For this review, use the dimensioned drawing (mm, ordinates from the lowest corner) and the shaded views. A direction names the side the tool comes from. Give positions to 0.01 mm unless a question says otherwise; leave off trailing zeros. Order: outer loops, then holes, each group sorted by start corner. A loop starts at its lowest first (then second) coordinate and runs counter-clockwise, first axis right, second up. Notation, with made-up numbers: (59, -20) -> (106, -20) arc R21 ccw to (106, 8) -> close; hole circle Ø7 at (84.25, 44). An arc over 180 degrees is marked (long way). Answer as a JSON object with one key per item and string values. Group by question number.
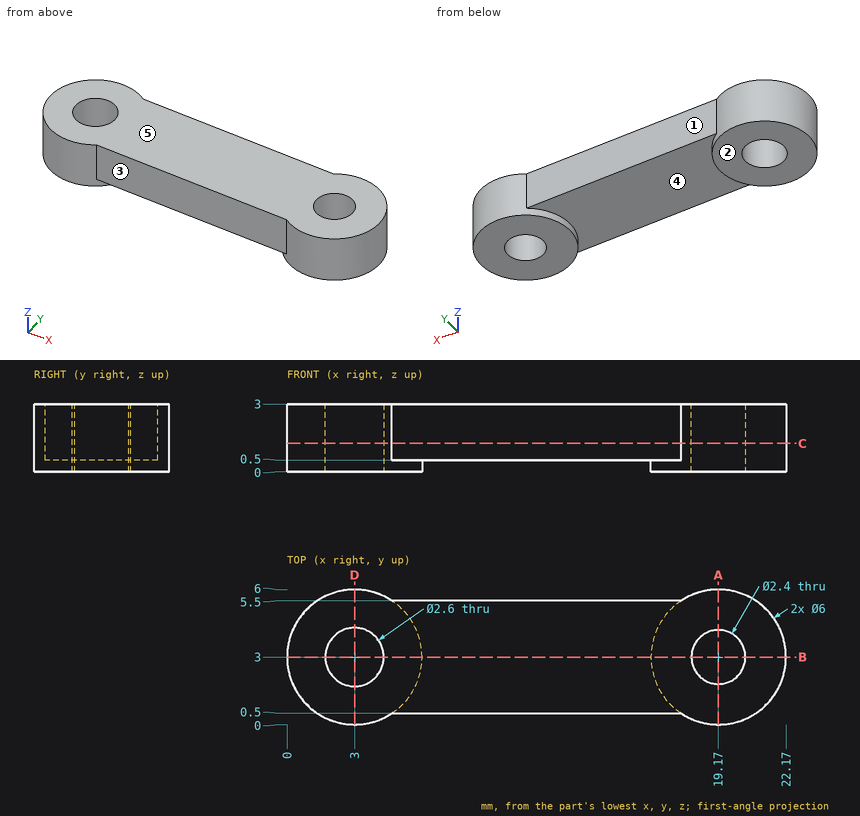
1. For probe 1 along X at (y, z) = (2, 1); probe 2 along X at (y, z) = (2.7, 1); probe 3 along Y at (x, z) = (3, 2.2), list the stretches that pass through material, from the lowest coordinate up. Write a range as [from, to].
2. Draft analysis for pull direction X (two halves, no side actions). For the marked faces 4 and 5, state which applies: pulls with the +X half, pulls with the -X half, needs draft (parallel to the pull), parting line crosses it, or undercut.
3. Take a section at D-D on x = 3. Give the boundary of the cut face in (y, z).
4. Take a section at A-A on x = 19.17. Give the boundary of the cut face in (y, z), plus the area to 3 significant figures.
5. Machinability: for the marked faces 1, 2 and 3, which of the approach directions +Z, -Z, +X, -X, +Y, -Y give a long, thin tool a straight path to every point of the face, cutting with its end or side? Answer none if there is none.
6. Take a section at C-C on z = 1.25. Give the boundary of the cut face in (x, y), plus the area to 3 significant figures.
7. Take a section at B-B on y = 3. Give the boundary of the cut face in (x, z).
8. For pin 1 (1.5 mm diameter, centred on x = 12.5, z = 2.5, fed in from +Y); pin 2 (2 mm diameter, centred on x = 11, y = 5.5, fed in from -Z), all flat-tipped, find the tip position at first contact; note any pin that passes through.
Checks:
{
 "1": {"probe 1": "x = [0.17, 2.17], [3.83, 18.51], [19.83, 22]", "probe 2": "x = [0.02, 1.74], [4.26, 18.01], [20.33, 22.15]", "probe 3": "y = [0, 1.7], [4.3, 6]"},
 "2": {"face 4": "undercut", "face 5": "needs draft"},
 "3": {"outline": "(0, 0) -> (1.7, 0) -> (1.7, 3) -> (0, 3) -> close; (4.3, 0) -> (6, 0) -> (6, 3) -> (4.3, 3) -> close"},
 "4": {"outline": "(0, 0) -> (1.8, 0) -> (1.8, 3) -> (0, 3) -> close; (4.2, 0) -> (6, 0) -> (6, 3) -> (4.2, 3) -> close", "area": "10.8 mm2"},
 "5": {"face 1": "+Z, -Z, +Y", "face 2": "-Z, +X, -X, +Y, -Y", "face 3": "+Z, -Z, -Y"},
 "6": {"outline": "(4.66, 0.5) -> (17.51, 0.5) arc R3 ccw (long way) to (17.51, 5.5) -> (4.66, 5.5) arc R3 ccw (long way) to start; hole circle Ø2.6 at (3, 3); hole circle Ø2.4 at (19.17, 3)", "area": "102 mm2"},
 "7": {"outline": "(0, 0) -> (1.7, 0) -> (1.7, 3) -> (0, 3) -> close; (4.3, 0) -> (6, 0) -> (6, 0.5) -> (16.17, 0.5) -> (16.17, 0) -> (17.97, 0) -> (17.97, 3) -> (4.3, 3) -> close; (20.37, 0) -> (22.17, 0) -> (22.17, 3) -> (20.37, 3) -> close"},
 "8": {"pin 1": "stops at y = 5.5", "pin 2": "stops at z = 0.5"}
}
